Autodesk Inventor part; units mm, degrees
ref_plane "YZ Plane" through (0, 0, 0) normal (1, 0, 0) x (0, 1, 0)
ref_plane "XZ Plane" through (0, 0, 0) normal (0, 1, 0) x (-1, 0, 0)
ref_plane "XY Plane" through (0, 0, 0) normal (0, 0, 1) x (1, 0, 0)
sketch "Sketch1" plane through (0, 0, 0) normal (0, 0, 1) x (1, 0, 0)
  circle A0 centre (0, 0) radius 11
  dimension "d0" = 22
extrude "Extrusion1" add sketch "Sketch1" along normal blind 10
sketch "Sketch2" plane through (0, 0, 10) normal (0, 0, 1) x (1, 0, 0)
  circle A0 centre (0, 0) radius 11
  circle A1 centre (0, 0) radius 8
  circle A2 centre (-8, 0) radius 1
  circle A3 centre (0, 8) radius 1
  circle A4 centre (8, 0) radius 1
  circle A5 centre (0, -8) radius 1
  dimension "d3" = 16
  dimension "d4" = 2
  dimension "d5" = 2
  dimension "d6" = 2
  dimension "d7" = 2
extrude "Extrusion2" cut sketch "Sketch2" against normal blind 10 contours A1 A4 | A1 A4 | A3 A1 | A1 A3 | A5 A1 | A1 A5 | A2 A1 | A1 A2
sketch "Sketch3" plane through (0, 0, 10) normal (0, 0, 1) x (1, 0, 0)
  circle A0 centre (8, 0) radius 1
  circle A1 centre (0, -8) radius 1
  circle A2 centre (-8, 0) radius 1
  circle A3 centre (0, 8) radius 1
  circle A4 centre (0, 0) radius 11
extrude "Extrusion3" add sketch "Sketch3" along normal blind 3
properties part number "awesomespin"
Input: part model. Units: mm. Frame: model coordinates. Coordinates: 2 decimals unless noted, no trailing zeros. Order: outer loops, then holes, each group sorted by start corner. A loop starts at its lowest first (then second) coordinate and runs counter-clockwise, first axis right, second up. Notation, with made-up numbers: M 24,55 L 38,55 A31 cw 38,88 Z; hole C 7,-27.5 d11. An arc over 180 degrees is marked long. Answer as CSV lines item,"result".
1. First-contact query: P1, Ø1.2, axis at x = 8, y = 0, coming from the -Z side; P2, Ø6, axis at x = 8.5, z = 9, coming from the +Y side; P3, Ø3, axis at y = 3.5, z = 10.5, coming from the -X side; P4, Ø3, axis at x = 6.5, z = 10, coming from the -Y side. Flat tips, straight axial feed; report the tip coordinate or a pass-through.
Reported:
P1,"through"
P2,"y = 9.53"
P3,"x = -10.82"
P4,"y = -9.8"
2. Pull-direction query (X, two-part tool) for faces 1 (the cylindrical face through (-2.38, 10.74, 6.41)), 2 (the cylindrical face through (7.2, 0.6, 6.4)), 3 (the flat face through (0, 0, 13)), 4 (the cylindrical face through (-8.8, 0.6, 6.4)); classes: released by +X, released by -X, zero draft, split by the parting line, or undercut.
Reported:
face 1,"split by the parting line"
face 2,"undercut"
face 3,"zero draft"
face 4,"undercut"
3. Section A-A (x = 0). Return the cut outline in (y, z).
Reported:
outline,"M -11,0 L -9,0 L -9,13 L -11,13 Z; M -7,0 L 7,0 L 7,13 L -7,13 Z; M 9,0 L 11,0 L 11,13 L 9,13 Z"
4. Section C-C (z = 2.25). Return the cut outline in (x, y), then the cut area to 3 significant figures.
Reported:
outline,"C 0,0 d22; hole C -8,0 d2; hole C 0,-8 d2; hole C 0,8 d2; hole C 8,0 d2"
area,"368 mm2"
5. Section D-D (x = -8). Return the cut outline in (y, z).
Reported:
outline,"M -7.55,0 L -1,0 L -1,13 L -7.55,13 Z; M 1,0 L 7.55,0 L 7.55,13 L 1,13 Z"
6. Material intervals for line 1 (Y direction, x = 0, z = 5.5); line 2 (Y direction, x = 0.75, z = 2.25); line 3 (Y direction, x = 8, z = 9.5), sorted ascending. Write a range as from..to.
Reported:
line 1,"-11..-9, -7..7, 9..11"
line 2,"-10.97..-8.66, -7.34..7.34, 8.66..10.97"
line 3,"-7.55..-1, 1..7.55"
